Part model, mm, in its own coordinate system. A direction names the side the tool comes from. Round coordinates to 2 decimals unless told otherwise and drop trailing zeros. Loops run counter-clockwise (first coordinate to the right, second up) from the corner with the lowest first, then second, coordinate; pieces in that order, holes last.
(1) Probe probe 1 along Y at (x, z) = (-11.5, 10); probe 2 along X at (y, z) = (-0.45, -14.75); probe 3 along Y at (x, z) = (8, 9.5). List the from-to ranges inside material, lowest first.
(2) Tool access for faces 4 (the face through (12, 0, 0)), 5 (the face through (-2.75, -8.66, -8.75)): list every direction of +Z, -Z, +X, -X, +Y, -Y with a clear straight run to the whole face (end or side of a thin tool).
(3) Flat gauge pins, fed straight in: pin 1 (3 mm diameter, centred on x = -13.5, z = 5.5, fed in from -Y); pin 2 (5.5 mm diameter, centred on x = 0, z = -14.75, fed in from +Y); pin 3 (8 mm diameter, centred on x = 9.5, z = 3.5, fed in from -Y); pin 4 (3 mm diameter, centred on x = -12.77, z = 7.37, fed in from +Y). Where does each tip first touch, or does it go through?
(4) Cut at D-D on y = -8.5. List the corners of the cut face in (x, z), then the cut area to 3 significant figures.
(5) Cut at B-B on z = 0. List the corners of the cut face in (x, y), then the cut area to 3 significant figures.
(6) Cut at A-A on x = 0. List the corners of the cut face in (y, z), then the cut area to 3 significant figures.
(7) Mould opens along X. For faces 1 (the face through (13.96, -0.99, 6.09)), 2 (the face through (-10.8, -2, 6.8)), 3 (the face through (7.3, 5.16, -3.8)) say: +X half, -X half, draft (parallel to the pull), parting line (faces both ways), or undercut.
(8) Cut at C-C on z = -14.75. List the corners of the cut face in (x, y), then the cut area to 3 significant figures.
from build123d import *

# Parameters (mm, degrees)
ESQUISSE3_R                  = 1.75
ENL_V_MAT_EXTRU_1_DEPTH      = 29.583211856
R_P_TITION_CIRCULAIRE1_COUNT = 3


with BuildPart() as part:
    # Esquisse1 → R_volution1 (revolve)
    with BuildSketch(Plane.XY, mode=Mode.PRIVATE) as r_volution1_sk:
        Polygon((0, 0), (0, 9), (8, 9), (8, 5.5), (11.69, 0), (18, 0), (18, -2), (12.5, -2), (9, -9), (0, -9), align=None)
    revolve(r_volution1_sk.sketch.rotate(Axis((0, 0, 0), (0, 1, 0)), 90), axis=Axis((0, 0, 0), (0, 1, 0)))

    # Esquisse2 → R_volution2 (revolve)
    with BuildSketch(Plane.XY):
        with BuildLine():
            Line((0, 7), (0, -13))
            ThreePointArc((0, -13), (10, -3), (0, 7))
        make_face()
    revolve(axis=Axis((0, 7, 0), (0, -1, 0)))

    # Esquisse3 → Enl_v. mat.-Extru.1 (cut, through all)
    with BuildSketch(Plane(origin=(0, 0, 0), x_dir=(1, 0, 0), z_dir=(0, 1, 0))):
        with Locations(Location((0, 14.75, 0), (0, 0, 270))):
            Circle(ESQUISSE3_R)
    enl_v_mat_extru_1 = extrude(amount=-ENL_V_MAT_EXTRU_1_DEPTH, mode=Mode.SUBTRACT)

    # R_p_tition circulaire1: Enl_v. mat.-Extru.1 ×3 about axis
    r_p_tition_circulaire1_axis = Axis((0, 0, 0), (0, 1, 0))
    for i in range(1, R_P_TITION_CIRCULAIRE1_COUNT):
        add(enl_v_mat_extru_1.rotate(r_p_tition_circulaire1_axis, i * 360 / R_P_TITION_CIRCULAIRE1_COUNT), mode=Mode.SUBTRACT)


solid = part.part
Final values:
1. probe 1: y = -2 to 0
1. probe 2: x = -10.32 to -1.75, 1.75 to 10.32
1. probe 3: y = -2.16 to 0
2. face 4: +Y
2. face 5: -Y
3. pin 1: stops at y = -2
3. pin 2: stops at y = 0
3. pin 3: stops at y = -10.91
3. pin 4: passes through
4. outline: circle Ø18.5 at (0, 0)
4. area: 269 mm2
5. outline: (-18, -2) - (-12.5, -2) - (-9, -9) - (-8, -9) arc R10 ccw to (8, -9) - (9, -9) - (12.5, -2) - (18, -2) - (18, 0) - (11.69, 0) - (8, 5.5) - (8, 9) - (-8, 9) - (-8, 5.5) - (-11.69, 0) - (-18, 0) - close
5. area: 432 mm2
6. outline: (-9, -9) - (-2, -12.5) - (-2, -13) - (0, -13) - (0, -11.69) - (5.5, -8) - (9, -8) - (9, 8) - (5.5, 8) - (0, 11.69) - (0, 18) - (-2, 18) - (-2, 12.5) - (-9, 9) - (-9, 8) arc R10 ccw to (-9, -8) - close; (-2, -18) - (0, -18) - (0, -16.5) - (-2, -16.5) - close
6. area: 425 mm2
7. face 1: undercut
7. face 2: draft
7. face 3: parting line
8. outline: (-10.32, -2) - (-1.75, -2) - (-1.75, 0) - (-10.32, 0) - close; (1.75, -2) - (10.32, -2) - (10.32, 0) - (1.75, 0) - close
8. area: 34.3 mm2
